Work out the finished part from the listing and answer in its coordinate system (mm). Coordinates: 2 decimals unless noted, no trailing zeros. Loops run counter-clockwise (first coordinate to the right, second up) from the corner with the lowest first, then second, coordinate; pieces in that order, holes last. Notation, with made-up numbers: (37, 88.5) -> (53, 88.5) arc R26 cw to (53, 122.5) -> close; hole circle Ø9 at (73.5, 50). An arc over 180 degrees is marked (long way). One line per question, with ' | ' between items.
```python
from build123d import *

# Parameters (mm, degrees)
SKETCH1_R           = 2.4892
BOSS_EXTRUDE1_DEPTH = 3.175


with BuildPart() as part:
    # Sketch1 → Boss-Extrude1 (new body)
    with BuildSketch(Plane(origin=(0, 0, 0), x_dir=(1, 0, 0), z_dir=(0, 1, 0))):
        Polygon((139.7, 0), (-139.7, 0), (-139.7, 25.4), (-101.6, 25.4), (-101.6, 150.6728), (27.94, 150.6728), (27.94, 25.4), (76.2, 25.4), (76.2, 76.2), (101.6, 76.2), (101.6, 25.4), (139.7, 25.4), align=None)
        with Locations((-127, 12.7)):
            Circle(SKETCH1_R, mode=Mode.SUBTRACT)
        with Locations((-88.9, 38.1)):
            Circle(SKETCH1_R, mode=Mode.SUBTRACT)
        with Locations((-88.9, 63.5)):
            Circle(SKETCH1_R, mode=Mode.SUBTRACT)
        with Locations((-79.375, 131.6228)):
            Circle(SKETCH1_R, mode=Mode.SUBTRACT)
        with Locations((-79.375, 106.2228)):
            Circle(SKETCH1_R, mode=Mode.SUBTRACT)
        with Locations((8.89, 106.2228)):
            Circle(SKETCH1_R, mode=Mode.SUBTRACT)
        with Locations((8.89, 131.6228)):
            Circle(SKETCH1_R, mode=Mode.SUBTRACT)
        with Locations((88.9, 63.5)):
            Circle(SKETCH1_R, mode=Mode.SUBTRACT)
        with Locations((88.9, 38.1)):
            Circle(SKETCH1_R, mode=Mode.SUBTRACT)
        with Locations((-101.6, 12.7)):
            Circle(SKETCH1_R, mode=Mode.SUBTRACT)
        with Locations((-76.2, 12.7)):
            Circle(SKETCH1_R, mode=Mode.SUBTRACT)
        with Locations((-50.8, 12.7)):
            Circle(SKETCH1_R, mode=Mode.SUBTRACT)
        with Locations((-25.4, 12.7)):
            Circle(SKETCH1_R, mode=Mode.SUBTRACT)
        with Locations((0, 12.7)):
            Circle(SKETCH1_R, mode=Mode.SUBTRACT)
        with Locations((25.4, 12.7)):
            Circle(SKETCH1_R, mode=Mode.SUBTRACT)
        with Locations((50.8, 12.7)):
            Circle(SKETCH1_R, mode=Mode.SUBTRACT)
        with Locations((76.2, 12.7)):
            Circle(SKETCH1_R, mode=Mode.SUBTRACT)
        with Locations((101.6, 12.7)):
            Circle(SKETCH1_R, mode=Mode.SUBTRACT)
        with Locations((127, 12.7)):
            Circle(SKETCH1_R, mode=Mode.SUBTRACT)
    extrude(amount=BOSS_EXTRUDE1_DEPTH)


solid = part.part
```
1) Find section C-C (z = -86.5). Write down the section's boundary in (x, y) (3 decimals).
Check values:
outline: (-101.6, 0) -> (27.94, 0) -> (27.94, 3.175) -> (-101.6, 3.175) -> close
2) Find section A-A (y = 0.85). State how many separate pieces and enclosed holes the cut face has, plus the area to 3 significant figures.
Check values:
separate pieces: 1 | enclosed holes: 19 | area: 24,200 mm^2
3) The mould has two halves that part along X. Classify faces 1 (the face through (129.374, 1.565, -13.448)), 2 (the face through (-29, 0, -60)), 3 (the face through (53.174, 1.565, -13.448)): released by +X, released by -X, zero draft, split by the parting line, or undercut.
Check values:
face 1: undercut | face 2: zero draft | face 3: undercut
4) Flat-ended cylindrical pins translate along their axes: pin 1 (1.6 mm diameter, centred on y = 1, z = -67, fed in from -X); pin 2 (2 mm diameter, centred on x = -32, z = -21, fed in from -Y); pin 3 (1 mm diameter, centred on x = 56.5, y = 1.5, fed in from -Z); pin 4 (1.6 mm diameter, centred on x = 93, y = 1, fed in from -Z). Find the tip coordinate at first contact, or state that the pin passes through.
Check values:
pin 1: stops at x = -101.6 | pin 2: stops at y = 0 | pin 3: stops at z = -25.4 | pin 4: stops at z = -76.2
5) Find the intervals of material crossed by line 1 along X through (y, z) = (0.75, -63.5); line 2 along X through (y, z) = (3.05, -33); line 3 along Z through (x, y) = (-50.8, 1.2), in increasing order.
Check values:
line 1: x = -101.6 to -91.39, -86.41 to 27.94, 76.2 to 86.41, 91.39 to 101.6 | line 2: x = -101.6 to 27.94, 76.2 to 101.6 | line 3: z = -150.67 to -15.19, -10.21 to 0
6) Find section B-B (x = -120). Write down the section's boundary in (y, z) (3 decimals), plus the area to 3 significant figures.
Check values:
outline: (0, -25.4) -> (3.175, -25.4) -> (3.175, 0) -> (0, 0) -> close | area: 80.6 mm^2
